Design review of the part built by this model. Coordinates are the model's own, in mm. A direction names the side the tool comes from. Coordinates: 2 decimals unless noted, no trailing zeros. Write each loop counter-clockwise with the first axis right and the second up, starting at its lowest first coordinate (ties: lowest second). Pieces come first, ordered by that corner, then holes.
Q1. For probe 1 along X at (y, z) = (2.25, -1.35) (3 decimals); probe 2 along Y at (x, z) = (0.5, -0.9) (3 decimals); probe 3 along X at (y, z) = (-1.5, 0.65) (3 decimals), list the stretches that pass through material, from the lowest coordinate up.
Q2. Machinability: for faces 1 (the cylindrical face through (2.19, -0.06, 1.31)), 2 (the flat face through (-4, 0, 1.588)), 3 (the flat face through (1.5, 0, -1)), which of the approach directions +Z, -Z, +X, -X, +Y, -Y give a long, thin tool a straight path to every point of the face, cutting with its end or side? Answer none if there is none.
Q3. Take a section at A-A (x = -0.75). Give the boundary of the cut face in (y, z) (1 decimal).
Q4. Mouldability with a two-part tool opening along Y and no side actions: class faces 4 (the cylindrical face through (0.04, 3.19, 1.31)), 5 (the flat face through (-4.675, 0, 0)), 6 (the flat face through (0, 5.675, 0)) as pulls with the +Y half, pulls with the -Y half, needs draft (parallel to the pull), parting line crosses it, or undercut.
Q5. Take a section at C-C (z = -0.15). Give the boundary of the cut face in (x, y) (3 decimals), and give its area (3 significant figures).
Q6. Insertion check: pin 1 (1 mm diameter, centred on x = -0.5, y = 3.5, fed in from +Z). The pin has a flat end and moves straight along its axis. Give the tip position at first contact, or say it passes through.
Q7. Take a section at B-B (y = -0.75). Give the boundary of the cut face in (x, z) (1 decimal), and give its area (3 significant figures).
Autodesk Inventor part; units mm, degrees
ref_plane "YZ Plane" through (0, 0, 0) normal (1, 0, 0) x (0, 1, 0)
ref_plane "XZ Plane" through (0, 0, 0) normal (0, 1, 0) x (-1, 0, 0)
ref_plane "XY Plane" through (0, 0, 0) normal (0, 0, 1) x (1, 0, 0)
sketch "Sketch1" plane through (0, 0, 0) normal (0, 0, 1) x (1, 0, 0)
  line L0 (-1.5, 2.5) -> (1.5, 2.5)
  line L1 (1.5, 2.5) -> (1.5, -2.5)
  line L2 (1.5, -2.5) -> (-1.5, -2.5)
  line L3 (-1.5, -2.5) -> (-1.5, 2.5)
  line L4 (-1.5, 2.5) -> (1.5, -2.5) construction
  line L5 (1.5, 2.5) -> (-1.5, -2.5) construction
  line L6 (4.675, 5.675) -> (-4.675, 5.675)
  line L7 (-4.675, 5.675) -> (-4.675, -5.675)
  line L8 (-4.675, -5.675) -> (4.675, -5.675)
  line L9 (4.675, -5.675) -> (4.675, 5.675)
  point P0 (0, 0)
  dimension "d0" = 3
  dimension "d1" = 5
  dimension "d2" = 3.175
extrude "Extrusion1" add sketch "Sketch1" along normal mid plane 3.175
fillet "Fillet1" radius 1.5875 2 edges at (0, 2.5, 1.5875) (0, -2.5, 1.5875)
fillet "Fillet2" radius 1.5875 2 edges at (-1.5, 0, 1.5875) (1.5, 0, 1.5875)
properties part number "Motor Fitting Test 2"
Response:
1. probe 1: x = -4.675 to -1.5, 1.5 to 4.675
1. probe 2: y = -5.675 to -2.5, 2.5 to 5.675
1. probe 3: x = -4.675 to -1.639, 1.639 to 4.675
2. face 1: +Z
2. face 2: +Z, +X, -X, +Y, -Y
2. face 3: +Z, -Z
3. outline: (-5.7, -1.6) - (-2.5, -1.6) - (-2.5, 0) arc R1.6 ccw to (-4.1, 1.6) - (-5.7, 1.6) - close; (2.5, -1.6) - (5.7, -1.6) - (5.7, 1.6) - (4.1, 1.6) arc R1.6 ccw to (2.5, 0) - close
4. face 4: undercut
4. face 5: needs draft
4. face 6: pulls with the +Y half
5. outline: (-4.675, -5.675) - (4.675, -5.675) - (4.675, 5.675) - (-4.675, 5.675) - close; hole (-1.5, -2.5) - (1.5, -2.5) - (1.5, 2.5) - (-1.5, 2.5) - close
5. area: 91.1 mm2
6. pin 1: stops at z = 1.59
7. outline: (-4.7, -1.6) - (-1.5, -1.6) - (-1.5, 0) arc R1.6 ccw to (-3.1, 1.6) - (-4.7, 1.6) - close; (1.5, -1.6) - (4.7, -1.6) - (4.7, 1.6) - (3.1, 1.6) arc R1.6 ccw to (1.5, 0) - close
7. area: 19.1 mm2
